from build123d import *

# Parameters (mm, degrees)
SKETCH1_R                   = 1.575
BOSS_EXTRUDE1_DEPTH         = 3.15
BOSS_EXTRUDE1_DEPTH_BACK    = 3.15
M2X0_25_TAPPED_HOLE1_D      = 1.75
M2X0_25_TAPPED_HOLE1_DEPTH  = 1.675
M2X0_25_TAPPED_HOLE2_REACH  = 21.046
M2X0_25_TAPPED_HOLE2_BORE_R = 0.875


with BuildPart() as part:
    # Sketch1 → Boss-Extrude1 (new, two sides)
    with BuildSketch(Plane(origin=(0, 0, 0), x_dir=(1, 0, 0), z_dir=(0, 1, 0))) as boss_extrude1_sk:
        with BuildLine():
            Line((-7.575, 3.25), (-9.25, 3.25))
            Line((-9.25, 3.25), (-9.25, -3.25))
            Line((-9.25, -3.25), (9.25, -3.25))
            Line((9.25, -3.25), (9.25, 3.25))
            Line((9.25, 3.25), (-3.76833041, 3.25))
            Line((-3.76833041, 3.25), (-3.76833041, 1.875))
            Line((-3.76833041, 1.875), (-1.7, 1.875))
            ThreePointArc((-1.7, 1.875), (0.175, 0), (-1.7, -1.875))
            Line((-1.7, -1.875), (-5.7, -1.875))
            ThreePointArc((-5.7, -1.875), (-7.025825215, -1.325825215), (-7.575, 0))
            Line((-7.575, 0), (-7.575, 3.25))
        make_face()
        with Locations(Location((5.55, 0, 0), (0, 0, 270))):
            Circle(SKETCH1_R, mode=Mode.SUBTRACT)
    extrude(amount=BOSS_EXTRUDE1_DEPTH)
    extrude(boss_extrude1_sk.sketch, amount=-BOSS_EXTRUDE1_DEPTH_BACK)

    # M2x0.25 Tapped Hole1
    with Locations(Plane.ZY.offset(9.25)):
        with Locations((0, 0)):
            Hole(M2X0_25_TAPPED_HOLE1_D / 2, depth=M2X0_25_TAPPED_HOLE1_DEPTH)

    # M2x0.25 Tapped Hole2 bore → M2x0.25 Tapped Hole2 (cut, up to next)
    with BuildSketch(Plane(origin=(9.25, 0, 0), x_dir=(0, 0, -1), z_dir=(1, 0, 0)), mode=Mode.PRIVATE) as m2x0_25_tapped_hole2_sk1:
        Circle(M2X0_25_TAPPED_HOLE2_BORE_R)
    m2x0_25_tapped_hole2_tool1 = extrude(m2x0_25_tapped_hole2_sk1.sketch, amount=-M2X0_25_TAPPED_HOLE2_REACH, mode=Mode.PRIVATE) & part.part
    add(m2x0_25_tapped_hole2_tool1.solids().sort_by_distance((9.25, 0, 0))[0], mode=Mode.SUBTRACT)


solid = part.part
Part model, mm, in its own coordinate system. A direction names the side the tool comes from. Coordinates: 2 decimals unless noted, no trailing zeros. Loops run counter-clockwise (first coordinate to the right, second up) from the corner with the lowest first, then second, coordinate; pieces in that order, holes last. Notation, with made-up numbers: (34, 73.25) -> (82, 73.25) arc R24 ccw to (82, 89.25) -> close; hole circle Ø6 at (62.25, 44.5). An arc over 180 degrees is marked (long way). Use a Markdown table: item, result. Add a question column.
Item 1: Which spindle directions (+Z, -Z, +X, -X, +Y, -Y) get a long thin tool onto all of the face, cutting with end or side? Do faces 1 (the flat face through (-4, 0, 1.875)), 2 (the cylindrical face through (-8.401, -0.335, -0.808)), 3 (the flat face through (-3.768, 0, -3)), 4 (the cylindrical face through (8.072, 0.038, 0.874)). Say none if no direction does.
Item 2: Band-saw the part on A-A on x = 5.55. Write the cut outline in (y, z) (3 decimals).
Item 3: Probe probe 1 along X at (y, z) = (2.5, 0) (3 decimals); probe 2 along X at (y, z) = (-1, -2.5) (3 decimals); probe 3 along Z at (x, y) = (-2.75, -2) (3 decimals). List the from-to ranges inside material, lowest first.
Item 4: Band-saw the part on D-D on z = -1.25. Write the cut outline in (x, y) (3 decimals), plus the area to 3 significant figures.
Item 5: Band-saw the part on C-C on y = -2.25. Write the cut outline in (x, z) (3 decimals), plus the area to 3 significant figures.
Item 6: Band-saw the part on B-B on y = 0. Write the cut outline in (x, z) (3 decimals).
Item 7: Pull direction Z, two halves, no side cores. Call faces 5 (the cylindrical face through (4.012, 0.044, -0.341)), 6 (the flat face through (-7.575, 0, -2)), 7 (the cylindrical face through (-7.01, 0.04, 1.34)): +Z half, -Z half, draft (parallel to the pull), parting line (faces both ways), or undercut.
Geometry says:
| question | item | result |
|---|---|---|
| 1 | face 1 | +Y, -Y |
| 1 | face 2 | -X |
| 1 | face 3 | -Z, +Y, -Y |
| 1 | face 4 | +X |
| 2 | outline | (-3.15, -3.25) -> (3.15, -3.25) -> (3.15, -1.575) -> (-3.15, -1.575) -> close; (-3.15, 1.575) -> (3.15, 1.575) -> (3.15, 3.25) -> (-3.15, 3.25) -> close |
| 3 | probe 1 | -9.25 to -7.575, 0.175 to 3.975, 7.125 to 9.25 |
| 3 | probe 2 | -9.25 to -7.575, -3.768 to 9.25 |
| 3 | probe 3 | -3.25 to -1.875, 1.875 to 3.25 |
| 4 | outline | (-9.25, -3.15) -> (-7.575, -3.15) -> (-7.575, 3.15) -> (-9.25, 3.15) -> close; (-0.302, -3.15) -> (4.592, -3.15) -> (4.592, 3.15) -> (-0.302, 3.15) -> close; (6.508, -3.15) -> (9.25, -3.15) -> (9.25, 3.15) -> (6.508, 3.15) -> close |
| 4 | area | 58.7 mm² |
| 5 | outline | (-9.25, -3.25) -> (-7.575, -3.25) -> (-7.575, 0) arc R1.875 cw to (-5.7, 1.875) -> (-1.7, 1.875) arc R1.875 cw to (-1.7, -1.875) -> (-3.768, -1.875) -> (-3.768, -3.25) -> (9.25, -3.25) -> (9.25, 3.25) -> (-9.25, 3.25) -> close; hole circle Ø3.15 at (5.55, 0) |
| 5 | area | 80.4 mm² |
| 6 | outline | (-9.25, -3.25) -> (-7.575, -3.25) -> (-7.575, -0.875) -> (-9.25, -0.875) -> close; (-9.25, 0.875) -> (-7.575, 0.875) -> (-7.575, 0) arc R1.875 cw to (-5.7, 1.875) -> (-1.7, 1.875) arc R1.875 cw to (-1.7, -1.875) -> (-3.768, -1.875) -> (-3.768, -3.25) -> (9.25, -3.25) -> (9.25, -0.875) -> (6.86, -0.875) arc R1.575 cw (long way) to (6.86, 0.875) -> (9.25, 0.875) -> (9.25, 3.25) -> (-9.25, 3.25) -> close |
| 7 | face 5 | undercut |
| 7 | face 6 | draft |
| 7 | face 7 | -Z half |
